Autodesk Inventor part; units mm, degrees
sketch "Sketch1" plane through (0, 0, 0) normal (0, 0, 1) x (1, 0, 0)
  circle A0 centre (0, 0) radius 50
  circle A1 centre (0, 0) radius 40
  dimension "d0" = 100
  dimension "d1" = 80
extrude "Extrusion1" add sketch "Sketch1" against normal blind 400
ref_plane "Work Plane1" through (0, 0, -400) normal (0, 0, -1) x (-1, 0, 0)
sketch "Sketch2" plane through (0, 0, -400) normal (0, 0, -1) x (-1, 0, 0)
  circle A0 centre (0, 0) radius 50
  circle A1 centre (0, 0) radius 40
  line L0 (0, 0) -> (0, 50)
sketch "Sketch3" plane through (0, 0, 0) normal (0, 1, 0) x (-1, 0, 0)
  point P0 (0, 0)
sketch "Sketch4" plane through (0, 0, 0) normal (0, 1, 0) x (-1, 0, 0)
  line L0 (70, -400) -> (-70, -400)
  line L1 (-50, -400) -> (50, -400)
  circle A0 centre (0, -400) radius 40
  circle A1 centre (0, -400) radius 50
  point P0 (0, 0)
  point P1 (40, -400)
  point P2 (-40, -400)
  dimension "d5" = 80
  dimension "d6" = 100
sketch "Sketch6" plane through (0, 0, 0) normal (0, 1, 0) x (-1, 0, 0)
  point P0 (0, 0)
sketch "Sketch7" plane through (0, 0, 0) normal (0, 1, 0) x (-1, 0, 0)
  line L0 (-40, -400) -> (-40, -400)
  circle A0 centre (0, -400) radius 40
  line L1 (-50, -400) -> (-50, -400)
  circle A1 centre (0, -400) radius 50
  point P0 (0, 0)
  point P1 (50, -400)
  point P2 (40, -400)
ref_plane "Work Plane4" through (50, 0, -400) normal (0, 0.7071, -0.7071) x (-1, 0, 0)
split "Split2" plane through (50, 0, -400) removes the side toward (0, 0.7071, -0.7071)
extrude "Extrusion3" add sketch "Sketch7" along normal blind 110
revolve "Revolution2" add sketch "Sketch4" angle 90 about axis through (0, 0, -400) along (-1, 0, 0) picked at (-46.3464, -403.2515) contours A1 L0 A0
ref_plane "Work Plane5" through (0, 110, -400) normal (0, 1, 0) x (1, 0, 0)
properties part number "Z2" material "Steel, Alloy"
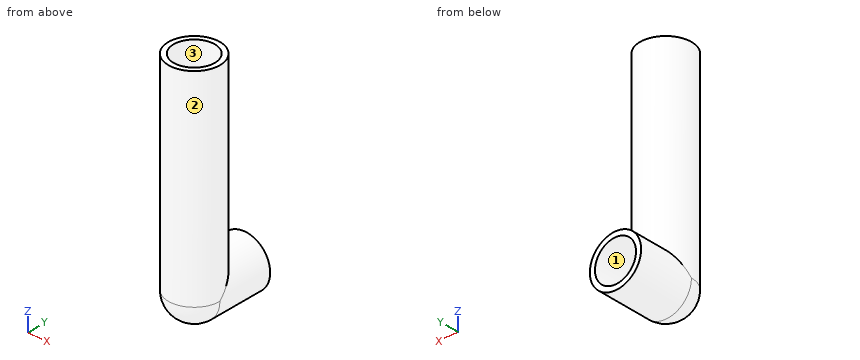
Verification items for the finished model (mm, model axes). Face numbers are marked on the shaded views. Give positions to 0.01 mm unless a question says otherwise; leave off trailing zeros. Order: outer loops, then holes, each group sorted by start corner. A loop starts at its lowest first (then second) coordinate and runs counter-clockwise, first axis right, second up. Notation, with made-up numbers: M 37,60 L 85,60 A22 cw 85,80 Z; hole C 59.25,66 d8. An arc over 180 degrees is marked long. Return JSON: item names as keys, results as strings. Group by question number.
1) Section check B-B on y = 83. Record the cut outline in (x, z).
2) Section check D-D on z = -112. Record the cut outline in (x, y), and give its area (3 significant figures).
3) Scan lines: line 1 (X direction, y = 0, z = -296); line 2 (Z direction, x = 0, y = 75). Record each from-to range of solid material in increasing order.
4) Section check C-C on z = -385.5. Record the cut outline in (x, y).
5) Mould release check, pull along X, two halves, no side actions. Record for the marked faces 1, 2 and 3: pulls with the +X half, pulls with the -X half, needs draft (parallel to the pull), parting line crosses it, or undercut.
6) Section check A-A on x = 0. Record the cut outline in (y, z).
7) Go/stop test with flat-tipped pins: pin 1 Ø10 at (x, z) = (32.5, -224.5) entering from +Y; pin 2 Ø8 at (x, z) = (-19, -194.5) entering from +Y; pin 3 Ø25 at (x, z) = (18.5, -374.5) entering from -Y. Record where each tip stops, or that it passes through.
Answer block:
{
 "1": {"outline": "C 0,-400 d100; hole C 0,-400 d80"},
 "2": {"outline": "C 0,0 d100; hole C 0,0 d80", "area": "2,830 mm^2"},
 "3": {"line 1": "x = -50 to -40, 40 to 50", "line 2": "z = -450 to -440, -360 to -350"},
 "4": {"outline": "M -47.85,14.5 A50 ccw long 47.85,14.5 L 47.85,110 L 37.28,110 L 37.28,0 L 40,0 A40 cw -40,0 L -37.28,0 L -37.28,110 L -47.85,110 Z"},
 "5": {"face 1": "undercut", "face 2": "parting line crosses it", "face 3": "undercut"},
 "6": {"outline": "M -50,-400 A50 ccw 0,-450 L 110,-450 L 110,-440 L 0,-440 A40 cw -40,-400 L -40,0 L -50,0 Z; M 0,-360 L 110,-360 L 110,-350 L 50,-350 L 50,0 L 40,0 L 40,-350 L 0,-350 Z"},
 "7": {"pin 1": "stops at y = 41.76", "pin 2": "stops at y = 47.7", "pin 3": "stops at y = -49.64"}
}
